Verification items for the finished model (mm, model axes). A direction names the side the tool comes from. Round coordinates to 2 decimals unless told otherwise and drop trailing zeros. Write each loop counter-clockwise with the first axis right and the second up, starting at its lowest first coordinate (ties: lowest second). Pieces come first, ordered by that corner, then holes. Notation, with made-up numbers: M 57,58 L 62,58 A36 ccw 62,94 Z; hole C 13,24.5 d7. An arc over 180 degrees is marked long. One line per question, with ' | ' between items. Start each with the question number.
Q1. Cross-section at C-C (z = 190.5). Record the boundary of the cut face in (x, y) (3 decimals), then the cut area to 3 significant figures.
Q2. Thickness scan on line 1 along Y through (x, z) = (1, 190); line 2 along Z through (x, y) = (0, 1.25); line 3 along Z through (x, y) = (-3.5, -11.5). Record the ranges inside material, lowest first. Write a range as from..to.
Q3. Gauge pin test, flat end, axial feed: pin 1 (18.5 mm diameter, centred on x = -11.5, z = 90, fed in from +Y). Record the tip position at first contact, or that the pin passes through.
Q4. Cross-section at D-D (x = 10.5). State how many separate pieces and enclosed holes the cut face has, then the cut area to 3 significant figures.
Q5. Tool access check on faces 1 (the face through (0, 0, 203.2)), 2 (the face through (0, 6.35, 80)). Record the directions out of +Z, -Z, +X, -X, +Y, -Y that give a thin tool (end or side, any length) a straight path to the whole face; none if there is none.
Q6. Release check for a two-part mould opening along Y. For faces 3 (the face through (-0.436, -2.16, 34.972)), 4 (the face through (31.115, -3, 100)), 5 (the face through (0.44, 8.16, 163.19)) record: released by +Y, released by -Y, zero draft, split by the parting line, or undercut.
Q7. Cross-section at B-B (y = 4.25). Record the boundary of the cut face in (x, z) (3 decimals), then the cut area to 3 significant figures.
Q8. Cross-section at A-A (z = 12.7). Record the boundary of the cut face in (x, y) (3 decimals).
from build123d import *

# Parameters (mm, degrees)
SKETCH1_W               = 62.23
SKETCH1_H               = 25.4
BOSS_EXTRUDE1_DEPTH     = 203.2
F_3_8_CLEARANCE_HOLE1_D = 9.8044
F_1_2_CLEARANCE_HOLE1_D = 13.89126
SKETCH16_W              = 62.23
SKETCH16_H              = 165.1
CUT_EXTRUDE2_DEPTH      = 6.35
FILLET1_R               = 6.35
CHAMFER1_SIZE           = 2.54
F_1_4_CLEARANCE_HOLE1_D = 6.7564


with BuildPart() as part:
    # Sketch1 → Boss-Extrude1 (new body)
    with BuildSketch(Plane.XY):
        Rectangle(SKETCH1_W, SKETCH1_H)
    extrude(amount=BOSS_EXTRUDE1_DEPTH)

    # 3/8 Clearance Hole1 (through all)
    with Locations(Plane(origin=(0, 12.7, 0), x_dir=(1, 0, 0), z_dir=(0, 1, 0))):
        with Locations((0, -12.7), (0, -127)):
            Hole(F_3_8_CLEARANCE_HOLE1_D / 2)

    # 1/2 Clearance Hole1 (through all)
    with Locations(Plane(origin=(31.115, 0, 0), x_dir=(0, 0, -1), z_dir=(1, 0, 0))):
        with Locations((-190.5, 0)):
            Hole(F_1_2_CLEARANCE_HOLE1_D / 2)

    # Sketch16 → Cut-Extrude2 (cut)
    with BuildSketch(Plane.XZ.offset(-12.7)):
        with Locations((0, 82.55)):
            Rectangle(SKETCH16_W, SKETCH16_H)
    extrude(amount=CUT_EXTRUDE2_DEPTH, mode=Mode.SUBTRACT)

    # Fillet1
    fillet1_edges = [part.edges().sort_by_distance(p)[0] for p in [
        (0, 6.35, 165.1),
    ]]
    fillet(fillet1_edges, radius=FILLET1_R - 0.0001)  # a hair under: the kernel refuses the full size

    # Chamfer1
    chamfer1_edges = [part.edges().sort_by_distance(p)[0] for p in [
        (0, -12.7, 203.2),
        (0, 12.7, 203.2),
    ]]
    chamfer(chamfer1_edges, length=CHAMFER1_SIZE)

    # 1/4 Clearance Hole1 (through all)
    with Locations(Plane(origin=(31.115, 0, 0), x_dir=(0, 0, -1), z_dir=(1, 0, 0))):
        with Locations((-31.75, -3.175)):
            Hole(F_1_4_CLEARANCE_HOLE1_D / 2)


solid = part.part
Determined:
1) outline: M -31.115,-12.7 L 31.115,-12.7 L 31.115,-6.946 L -31.115,-6.946 Z; M -31.115,6.946 L 31.115,6.946 L 31.115,12.7 L -31.115,12.7 Z | area: 716 mm²
2) line 1: y = -12.7..-6.93, 6.93..12.7 | line 2: z = 0..7.8, 17.6..122.1, 131.9..183.67, 197.33..203.2 | line 3: z = 0..9.27, 16.13..123.57, 130.43..201.86
3) pin 1: stops at y = 6.35
4) separate pieces: 1 | enclosed holes: 2 | area: 3,930 mm²
5) face 1: +Z, +X, -X, +Y, -Y | face 2: -Z, +X, -X, +Y
6) face 3: undercut | face 4: zero draft | face 5: released by +Y
7) outline: M -31.115,0 L 31.115,0 L 31.115,185.006 L -31.115,185.006 Z; M -31.115,195.994 L 31.115,195.994 L 31.115,203.2 L -31.115,203.2 Z; hole C 0,12.7 d9.804; hole C 0,127 d9.804 | area: 11,800 mm²
8) outline: M -31.115,-12.7 L -4.902,-12.7 L -4.902,6.35 L -31.115,6.35 Z; M 4.902,-12.7 L 31.115,-12.7 L 31.115,6.35 L 4.902,6.35 Z
